Part model, mm, in its own coordinate system. A direction names the side the tool comes from. Round coordinates to 2 decimals unless told otherwise and drop trailing zeros. Loops run counter-clockwise (first coordinate to the right, second up) from the corner with the lowest first, then second, coordinate; pieces in that order, holes last.
1) Band-saw the part on A-A, the plane z = 35. Write the cut outline in (x, y).
2) Mould opens along Z. For faces 4 (the flat face through (0, 158, 35)), 5 (the flat face through (1, -6, 43.5)), 6 (the flat face through (-20, 29, 28)) say: +Z half, -Z half, draft (parallel to the pull), parting line (faces both ways), or undercut.
3) 3-axis set-ups, long thin cutter, end or side, ignore diameter. For faces 1 (the flat face through (1, -6, 26.5)), 2 (the cylindrical face through (0, 310, 25)), 3 (the flat face through (0, 142, 0)): which of +Z, -Z, +X, -X, +Y, -Y reach the whole face in a straight line?
4) Probe line 1 (X direction, y = 367.5, z = 35); line 2 (Z direction, x = 1, y = 95.5); line 3 (Y direction, x = -4, z = 28). List the from-to ranges inside material, lowest first.
5) Drop flat-ended pins along their axis: P1, Ø5, axis at x = -13, y = 400, coming from the -Z side; P2, Ø2, axis at y = 104, z = 33, coming from the +X side; P3, Ø17, axis at x = 8, z = -6, coming from the +Y side; P4, Ø5, axis at y = 364.5, z = 16, coming from the +X side. Give the stop position or say it passes through.
6) Band-saw the part on B-B, the plane y = 428. Write the cut outline in (x, z), then the cut area to 3 significant figures.
from build123d import *

# Parameters (mm, degrees)
EXTRUDE_1_DEPTH     = 58
SKETCH_2_R          = 20
EXTRUDE_7_DEPTH     = 78
SKETCH_3_R          = 14.5
EXTRUDE_8_DEPTH     = 400
SKETCH_4_R          = 10
CUT_EXTRUDE_1_DEPTH = 300
FILLET_2_R          = 3
FILLET_START        = -21
FILLET_3_DEPTH      = 77
FILLET_3_2_DEPTH    = 41
FILLET_3_3_ANGLE    = 180
FILLET_4_R          = 3
SKETCH_6_R          = 9
EXTRUDE_10_DEPTH    = 6
FILLET_5_R          = 3
FILLET_6_R          = 3
EXTRUDE_11_DEPTH    = 18
FILLET_7_R          = 2
SKETCH_9_R          = 3.25
CUT_EXTRUDE_2_DEPTH = 463.813407343


with BuildPart() as part:
    # 草图1 → 凸台-拉伸1 (new body)
    with BuildSketch(Plane(origin=(0, 0, 0), x_dir=(1, 0, 0), z_dir=(0, 1, 0))):
        with BuildLine():
            Line((20, 0), (20, -55))
            Line((20, -55), (-20, -55))
            Line((-20, -55), (-20, 0))
            ThreePointArc((-20, 0), (0, 20), (20, 0))
        make_face()
    extrude(amount=EXTRUDE_1_DEPTH)

    # 草图2 → 凸台-拉伸7 (add)
    with BuildSketch(Plane(origin=(0, 58, 0), x_dir=(1, 0, 0), z_dir=(0, 1, 0))):
        with Locations(Location((0, 0, 0), (0, 0, 180))):
            Circle(SKETCH_2_R)
    extrude(amount=EXTRUDE_7_DEPTH)

    # 草图3 → 凸台-拉伸8 (add)
    with BuildSketch(Plane(origin=(0, 58, 0), x_dir=(1, 0, 0), z_dir=(0, 1, 0))):
        with Locations(Location((0, -35, 0), (0, 0, 270))):
            Circle(SKETCH_3_R)
    extrude(amount=EXTRUDE_8_DEPTH)

    # 草图4 → 切除-拉伸1 (cut)
    with BuildSketch(Plane(origin=(0, 458, 0), x_dir=(1, 0, 0), z_dir=(0, 1, 0))):
        with Locations(Location((0, -35, 0), (0, 0, 270))):
            Circle(SKETCH_4_R)
    extrude(amount=-CUT_EXTRUDE_1_DEPTH, mode=Mode.SUBTRACT)

    # 圆角2
    # the kernel refuses this fillet: 3 mm, written as the material it takes off along each edge
    with BuildSketch(Plane(origin=(27.5, 58, 55), x_dir=(0, -1, 0), z_dir=(-1, 0, 0))) as fillet_2_piece_1:
        with BuildLine():
            CenterArc((FILLET_2_R, -FILLET_2_R), FILLET_2_R, 90, 90)
            Line((0, -FILLET_2_R), (0, 0))
            Line((0, 0), (FILLET_2_R, 0))
        make_face()
    extrude(amount=55, mode=Mode.SUBTRACT)
    with BuildSketch(Plane(origin=(20, 58, -12.75), x_dir=(0, -1, 0), z_dir=(0, 0, 1))) as fillet_2_piece_2_section:
        with BuildLine():
            CenterArc((FILLET_2_R, -FILLET_2_R), FILLET_2_R, 90, 90)
            Line((0, -FILLET_2_R), (0, 0))
            Line((0, 0), (FILLET_2_R, 0))
        make_face()
    fillet_2_piece_2 = extrude(amount=75.25, mode=Mode.PRIVATE)
    fillet_2_piece_2 = fillet_2_piece_2 - Plane(origin=(0, 58, 0), x_dir=(-1, 0, 0), z_dir=(0, -1, 0)) * Cylinder(20, 163, mode=Mode.PRIVATE)
    add(fillet_2_piece_2, mode=Mode.SUBTRACT)
    with BuildSketch(Plane(origin=(-20, 58, 62.5), x_dir=(1, 0, 0), z_dir=(0, 0, -1))) as fillet_2_piece_3_section:
        with BuildLine():
            CenterArc((FILLET_2_R, FILLET_2_R), FILLET_2_R, 180, 90)
            Line((0, FILLET_2_R), (0, 0))
            Line((0, 0), (FILLET_2_R, 0))
        make_face()
    fillet_2_piece_3 = extrude(amount=75.25, mode=Mode.PRIVATE)
    fillet_2_piece_3 = fillet_2_piece_3 - Plane(origin=(0, 58, 0), x_dir=(-1, 0, 0), z_dir=(0, -1, 0)) * Cylinder(20, 163, mode=Mode.PRIVATE)
    add(fillet_2_piece_3, mode=Mode.SUBTRACT)

    # 圆角3: read off the stored shape, not the designer's step
    # 圆角3 outline → 圆角3 (cut)
    with BuildSketch(Plane.XY.offset(FILLET_START)):
        with BuildLine():
            Line((20, 0), (20, 3))
            ThreePointArc((20, 3), (19.121320344, 0.878679656), (17, 0))
            Line((17, 0), (20, 0))
        make_face()
        with BuildLine():
            Line((-20, 0), (-17, 0))
            ThreePointArc((-17, 0), (-19.121320344, 0.878679656), (-20, 3))
            Line((-20, 3), (-20, 0))
        make_face()
    extrude(amount=FILLET_3_DEPTH, mode=Mode.SUBTRACT)

    # Fillet 3 2 outline → Fillet 3 2 (cut)
    with BuildSketch(Plane.YZ.offset(FILLET_START)):
        with BuildLine():
            ThreePointArc((0, 52), (0.878679656, 54.121320344), (3, 55))
            Line((3, 55), (0, 55))
            Line((0, 55), (0, 52))
        make_face()
    extrude(amount=FILLET_3_2_DEPTH, mode=Mode.SUBTRACT)

    # Fillet 3 3 outline → Fillet 3 3 (revolve, cut)
    with BuildSketch(Plane.XY):
        with BuildLine():
            ThreePointArc((20, 3), (19.121320344, 0.878679656), (17, 0))
            Line((17, 0), (20, 0))
            Line((20, 0), (20, 3))
        make_face()
    revolve(axis=Axis((0, 0, 0), (0, 1, 0)), revolution_arc=FILLET_3_3_ANGLE, mode=Mode.SUBTRACT)

    # 圆角4
    fillet_4_edges = [part.edges().sort_by_distance(p)[0] for p in [
        (20, 136, 0),
    ]]
    fillet(fillet_4_edges, radius=FILLET_4_R)

    # 草图6 → 凸台-拉伸10 (add)
    with BuildSketch(Plane(origin=(0, 136, 0), x_dir=(1, 0, 0), z_dir=(0, 1, 0))):
        with Locations(Location((0, 0, 0), (0, 0, 270))):
            Circle(SKETCH_6_R)
    extrude(amount=EXTRUDE_10_DEPTH)

    # 圆角5
    fillet_5_edges = [part.edges().sort_by_distance(p)[0] for p in [
        (0, 136, -9),
        (0, 142, -9),
    ]]
    fillet(fillet_5_edges, radius=FILLET_5_R - 0.0001)  # a hair under: the kernel refuses the full size

    # 圆角6
    fillet_6_edges = [part.edges().sort_by_distance(p)[0] for p in [
        (0, 458, 20.5),
    ]]
    fillet(fillet_6_edges, radius=FILLET_6_R)

    # 草图7 → 凸台-拉伸11 (add)
    with BuildSketch(Plane.XZ):
        with BuildLine():
            Line((-5.404550966, 43.5), (7.595449034, 43.5))
            ThreePointArc((7.595449034, 43.5), (9.009662596, 42.914213562), (9.595449034, 41.5))
            Line((9.595449034, 41.5), (9.595449034, 28.5))
            ThreePointArc((9.595449034, 28.5), (9.009662596, 27.085786438), (7.595449034, 26.5))
            Line((7.595449034, 26.5), (-5.404550966, 26.5))
            ThreePointArc((-5.404550966, 26.5), (-6.818764529, 27.085786438), (-7.404550966, 28.5))
            Line((-7.404550966, 28.5), (-7.404550966, 41.5))
            ThreePointArc((-7.404550966, 41.5), (-6.818764529, 42.914213562), (-5.404550966, 43.5))
        make_face()
    extrude(amount=EXTRUDE_11_DEPTH)

    # 圆角7
    fillet_7_edges = [part.edges().sort_by_distance(p)[0] for p in [
        (-6.818764529, -18, 42.914213562),
        (-7.404550966, -18, 35),
        (-6.818764529, -18, 27.085786438),
        (1.095449034, -18, 26.5),
        (9.009662596, -18, 27.085786438),
        (9.595449034, -18, 35),
        (9.009662596, -18, 42.914213562),
        (1.095449034, -18, 43.5),
    ]]
    fillet(fillet_7_edges, radius=FILLET_7_R)

    # 草图9 → 切除-拉伸2 (cut, through all)
    with BuildSketch(Plane.XY.offset(43.5)):
        with Locations((1.095449034, -9.5)):
            Circle(SKETCH_9_R)
    extrude(amount=-CUT_EXTRUDE_2_DEPTH, mode=Mode.SUBTRACT)


solid = part.part
Reported:
1. outline: (-20, 3) arc R3 ccw to (-17, 0) - (-7.4, 0) - (-7.4, -16) arc R2 ccw to (-5.4, -18) - (7.6, -18) arc R2 ccw to (9.6, -16) - (9.6, 0) - (17, 0) arc R3 ccw to (20, 3) - (20, 55) arc R3 ccw to (17, 58) - (14.5, 58) - (14.5, 455) arc R3 ccw to (11.5, 458) - (10, 458) - (10, 158) - (-10, 158) - (-10, 458) - (-11.5, 458) arc R3 ccw to (-14.5, 455) - (-14.5, 58) - (-17, 58) arc R3 ccw to (-20, 55) - close; hole circle Ø6.5 at (1.1, -9.5)
2. face 4: undercut
2. face 5: +Z half
2. face 6: draft
3. face 1: -Z, +X, -X, -Y
3. face 2: +Y
3. face 3: -Z, +X, -X, +Y
4. line 1: x = -14.5 to -10, 10 to 14.5
4. line 2: z = -19.97 to 19.97, 20.53 to 49.47
4. line 3: y = -17.94 to 158
5. P1: stops at z = 25
5. P2: stops at x = 14.47
5. P3: stops at y = 142
5. P4: passes through
6. outline: circle Ø29 at (0, 35); hole circle Ø20 at (0, 35)
6. area: 346 mm2
